Can you work these out from the model? Positions are in its coordinate system, mm. A direction names the side the tool comes from. Round coordinates to 2 decimals unless told otherwise and drop trailing zeros. Write each loop counter-clockwise with the first axis right and the second up, starting at its lowest first coordinate (ties: lowest second). Pieces come first, ordered by that corner, then holes. Notation, with made-up numbers: (23, 46) -> (29, 46) arc R15 ccw to (29, 50) -> close; hole circle Ø7 at (-34, 78). An arc over 180 degrees is marked (long way). Use CSV: the item, a comma, the result in double quotes.
```python
from build123d import *

# Parameters (mm, degrees)
EXTRUDE_451_DEPTH           = 3
SKETCH_505_W                = 3
SKETCH_505_H                = 16
EXTRUDE_763_DEPTH           = 20
CUT_EXTRUDE_1013_DEPTH      = 5
CUT_EXTRUDE_1013_DEPTH_BACK = 3
SKETCH_8_W                  = 3
SKETCH_8_H                  = 16
EXTRUDE_1404_DEPTH          = 20
CUT_EXTRUDE_1670_DEPTH      = 64
CUT_EXTRUDE_1670_DEPTH_BACK = 3
SKETCH_11_W                 = 56
SKETCH_11_H                 = 2.665153407
EXTRUDE_1980_DEPTH          = 7


with BuildPart() as part:
    # Sketch 219 → Extrude 451 (new body)
    with BuildSketch(Plane(origin=(0, 0, 0), x_dir=(1, 0, 0), z_dir=(0, 1, 0))):
        with BuildLine():
            Line((2, 0), (68, 0))
            ThreePointArc((68, 0), (69.414213562, 0.585786438), (70, 2))
            Line((70, 2), (70, 18))
            ThreePointArc((70, 18), (69.414213562, 19.414213562), (68, 20))
            Line((68, 20), (2, 20))
            ThreePointArc((2, 20), (0.585786438, 19.414213562), (0, 18))
            Line((0, 18), (0, 2))
            ThreePointArc((0, 2), (0.585786438, 0.585786438), (2, 0))
        make_face()
    extrude(amount=EXTRUDE_451_DEPTH)

    # Sketch 505 → Extrude 763 (add)
    with BuildSketch(Plane(origin=(0, 3, 0), x_dir=(1, 0, 0), z_dir=(0, 1, 0))):
        with Locations((5.5, 10)):
            Rectangle(SKETCH_505_W, SKETCH_505_H)
    extrude(amount=EXTRUDE_763_DEPTH)

    # Sketch 818 → Cut-Extrude 1013 (cut, two sides)
    with BuildSketch(Plane.ZY.offset(-4)) as cut_extrude_1013_sk:
        Polygon((-45.532064127, 82.064128255), (-16, 23), (-10, 11), (-4, 23), (25.532064127, 82.064128255), (25.532064127, 214.135534064), (-45.532064127, 214.135534064), align=None)
    extrude(amount=CUT_EXTRUDE_1013_DEPTH, mode=Mode.SUBTRACT)
    extrude(cut_extrude_1013_sk.sketch, amount=-CUT_EXTRUDE_1013_DEPTH_BACK, mode=Mode.SUBTRACT)

    # Эскиз8 → Extrude 1404 (add)
    with BuildSketch(Plane(origin=(31.408501121, 3, 2.625790974), x_dir=(1, 0, 0), z_dir=(0, 1, 0))):
        with Locations((33.091498879, 12.625790974)):
            Rectangle(SKETCH_8_W, SKETCH_8_H)
    extrude(amount=EXTRUDE_1404_DEPTH)

    # Эскиз10 → Cut-Extrude 1670 (cut, two sides)
    with BuildSketch(Plane(origin=(63, 0, 2.625790974), x_dir=(0, 0, 1), z_dir=(-1, 0, 0))) as cut_extrude_1670_sk:
        Polygon((-48.157855101, 82.064128255), (-18.625790974, 23), (-12.625790974, 11), (-6.625790974, 23), (22.906273154, 82.064128255), (22.906273154, 214.135534064), (-48.157855101, 214.135534064), align=None)
    extrude(amount=CUT_EXTRUDE_1670_DEPTH, mode=Mode.SUBTRACT)
    extrude(cut_extrude_1670_sk.sketch, amount=-CUT_EXTRUDE_1670_DEPTH_BACK, mode=Mode.SUBTRACT)

    # Эскиз11 → Extrude 1980 (add)
    with BuildSketch(Plane(origin=(0, 3, 0), x_dir=(1, 0, 0), z_dir=(0, 1, 0))):
        with Locations((35, 10.036015586)):
            Rectangle(SKETCH_11_W, SKETCH_11_H)
    extrude(amount=EXTRUDE_1980_DEPTH)


solid = part.part
```
Q1. Please list where these lines run through material, in increasing order: probe 1 along X at (y, z) = (18, -3.5); probe 2 along Y at (x, z) = (59.5, -15.5); probe 3 along Z at (x, y) = (7.5, 6.25).
Resolved:
probe 1,"x = 4 to 7, 63 to 66"
probe 2,"y = 0 to 3"
probe 3,"z = -11.37 to -8.7"
Q2. Suppose I cut it at A-A (y = 15). Write out the boundary of the cut face in (x, z), and give its area (3 significant figures).
Resolved:
outline,"(4, -18) -> (7, -18) -> (7, -12) -> (4, -12) -> close; (4, -8) -> (7, -8) -> (7, -2) -> (4, -2) -> close; (63, -18) -> (66, -18) -> (66, -12) -> (63, -12) -> close; (63, -8) -> (66, -8) -> (66, -2) -> (63, -2) -> close"
area,"72.0 mm^2"
Q3. On a 3-axis mill with a long thin cutter (end or side, diameter ignored), from which of +Z, -Z, +X, -X, +Y, -Y can I reach the whole of each face in a straight line? I mean faces 1 (the face through (64, 13, -18)), 2 (the face through (35, 6, -11.369)), 3 (the face through (5, 13, -2)), 4 (the face through (5, 17, -13)). Say none if no direction works.
Resolved:
face 1,"-Z, +X, -X, +Y"
face 2,"-Z, +Y"
face 3,"+Z, +X, -X, +Y"
face 4,"+X, -X, +Y"
Q4. Suppose I cut it at C-C (x = 22). Write out the boundary of the cut face in (y, z), and give its area (3 significant figures).
Resolved:
outline,"(0, -20) -> (3, -20) -> (3, -11.37) -> (10, -11.37) -> (10, -8.7) -> (3, -8.7) -> (3, 0) -> (0, 0) -> close"
area,"78.7 mm^2"
Q5. Suppose I cut it at D-D (y = 12). Write out the boundary of the cut face in (x, z), and give its area (3 significant figures).
Resolved:
outline,"(4, -18) -> (7, -18) -> (7, -10.5) -> (4, -10.5) -> close; (4, -9.5) -> (7, -9.5) -> (7, -2) -> (4, -2) -> close; (63, -18) -> (66, -18) -> (66, -10.5) -> (63, -10.5) -> close; (63, -9.5) -> (66, -9.5) -> (66, -2) -> (63, -2) -> close"
area,"90.0 mm^2"
Q6. Suppose I cut it at B-B (z = -17). Write out the boundary of the cut face in (x, y), and give its area (3 significant figures).
Resolved:
outline,"(0, 0) -> (70, 0) -> (70, 3) -> (66, 3) -> (66, 23) -> (63, 23) -> (63, 3) -> (7, 3) -> (7, 23) -> (4, 23) -> (4, 3) -> (0, 3) -> close"
area,"330 mm^2"
Q7. If we mould it in two halves opening along X, with no side actions, what happens to faces 5 (the face through (0, 1, -10)), 6 (the face through (63, 10.6, -9.9)), 7 (the face through (35, 1, 0))? For each: released by +X, released by -X, zero draft, split by the parting line, or undercut.
Resolved:
face 5,"released by -X"
face 6,"undercut"
face 7,"zero draft"
Q8. Will these pins go through, and if not, where does the flat tip stop? P1, Ø8, axis at y = 17.5, z = -7.5, coming from the +X side; P2, Ø3.5, axis at x = 35, y = 5, coming from the +Z side; P3, Ø2.5, axis at x = 64, y = 13, coming from the -Z side.
Resolved:
P1,"stops at x = 66"
P2,"stops at z = -8.7"
P3,"stops at z = -18"
